Design review of the part built by this model. Coordinates are the model's own, in mm. A direction names the side the tool comes from. Round coordinates to 2 decimals unless told otherwise and drop trailing zeros. Order: outer loops, then holes, each group sorted by start corner. A loop starts at its lowest first (then second) coordinate and runs counter-clockwise, first axis right, second up. Notation, with made-up numbers: (11.5, -18) - (69.5, -18) arc R22 ccw to (69.5, 11) - close; hole circle Ø1 at (17, 29.5). An arc over 180 degrees is marked (long way). Write item = value, one per line.
from build123d import *

# Parameters (mm, degrees)
SKETCH1_W                       = 45.72
SKETCH1_H                       = 60.96
BOSS_EXTRUDE1_DEPTH             = 6.35
SKETCH2_W                       = 7.8600046
SKETCH2_H                       = 60.96
BOSS_EXTRUDE2_DEPTH             = 20.955
LPATTERN1_COUNT                 = 3
LPATTERN1_PITCH                 = 17.018
SKETCH1_3_W                     = 45.72
SKETCH1_3_H                     = 60.96
BOSS_EXTRUDE3_DEPTH             = 2.54
CUT_EXTRUDE1_START              = 14.999995
SKETCH11_W                      = 60.96
SKETCH11_H                      = 14.3449802
CUT_EXTRUDE1_DEPTH              = 17.78
CUT_EXTRUDE2_DEPTH              = 62.358877312
SKETCH17_W                      = 45.72
SKETCH17_H                      = 60.96
BOSS_EXTRUDE4_DEPTH             = 6.985
SKETCH19_W                      = 29.9999908
SKETCH19_H                      = 60.96
BOSS_EXTRUDE5_DEPTH             = 1.0100056
CBORE_FOR_M5_SBHCS2_D           = 5.5
CBORE_FOR_M5_SBHCS2_CBORE_D     = 10.5
CBORE_FOR_M5_SBHCS2_CBORE_DEPTH = 2.75
CUT_EXTRUDE3_DEPTH              = 82.222264916
CUT_EXTRUDE3_DEPTH_BACK         = 82.222264916
SKETCH24_W                      = 5.08
SKETCH24_H                      = 45.72
CUT_EXTRUDE4_DEPTH              = 9.874000032


with BuildPart() as part:
    # Sketch1 → Boss-Extrude1 (new body)
    with BuildSketch(Plane(origin=(0, 0, 0), x_dir=(1, 0, 0), z_dir=(0, 1, 0))):
        Rectangle(SKETCH1_W, SKETCH1_H)
    extrude(amount=BOSS_EXTRUDE1_DEPTH)

    # Sketch2 → Boss-Extrude2 (add)
    with BuildSketch(Plane(origin=(0, 6.35, 0), x_dir=(1, 0, 0), z_dir=(0, 1, 0))):
        with Locations((-18.9299977, 0)):
            Rectangle(SKETCH2_W, SKETCH2_H)
        with Locations((18.9299977, 0)):
            Rectangle(SKETCH2_W, SKETCH2_H)
    extrude(amount=BOSS_EXTRUDE2_DEPTH)

    # Sketch7 → M2 Clearance Hole2 (revolve, cut)
    with BuildSketch(Plane(origin=(22.86, 10.16, 14.9171914), x_dir=(0, 0, -1), z_dir=(0, 1, 0))):
        Polygon((0, 0), (0, 46.441032743), (1.2, 45.72), (1.2, 0), align=None)
    m2_clearance_hole2 = revolve(axis=Axis((29.21, 10.16, 14.9171914), (-1, 0, 0)), mode=Mode.SUBTRACT)

    # LPattern1: M2 Clearance Hole2 ×3
    with Locations(*[(0, 0, -i * LPATTERN1_PITCH) for i in range(1, LPATTERN1_COUNT)]):
        add(m2_clearance_hole2, mode=Mode.SUBTRACT)

    # Sketch1<3> → Boss-Extrude3 (add)
    with BuildSketch(Plane(origin=(0, 0, 0), x_dir=(1, 0, 0), z_dir=(0, 1, 0))):
        Rectangle(SKETCH1_3_W, SKETCH1_3_H)
    extrude(amount=-BOSS_EXTRUDE3_DEPTH)

    # Sketch11 → Cut-Extrude1 (cut, symmetric)
    with BuildSketch(Plane.ZY.offset(-14.9999954).offset(CUT_EXTRUDE1_START)):
        with Locations((0, 20.1325099)):
            Rectangle(SKETCH11_W, SKETCH11_H)
    extrude(amount=CUT_EXTRUDE1_DEPTH, both=True, mode=Mode.SUBTRACT)

    # Sketch12 → Cut-Extrude2 (cut, through all)
    with BuildSketch(Plane(origin=(22.86, 0, 0), x_dir=(0, 0, -1), z_dir=(1, 0, 0))):
        with BuildLine():
            Line((13.105000048, 12.7), (30.48, 12.7))
            Line((30.48, 12.7), (30.48, 27.305))
            Line((30.48, 27.305), (25.661312206, 27.305))
            ThreePointArc((25.661312206, 27.305), (3.474748234, 33.679387055), (13.105000048, 12.7))
        make_face()
    extrude(amount=-CUT_EXTRUDE2_DEPTH, mode=Mode.SUBTRACT)

    # Sketch17 → Boss-Extrude4 (add)
    with BuildSketch(Plane.XZ.offset(2.54)):
        Rectangle(SKETCH17_W, SKETCH17_H)
    extrude(amount=BOSS_EXTRUDE4_DEPTH)

    # Sketch19 → Boss-Extrude5 (add)
    with BuildSketch(Plane(origin=(0, 6.35, 0), x_dir=(1, 0, 0), z_dir=(0, 1, 0))):
        Rectangle(SKETCH19_W, SKETCH19_H)
    extrude(amount=BOSS_EXTRUDE5_DEPTH)

    # CBORE for M5 SBHCS2 (through all)
    with Locations(Plane(origin=(0, 7.3600056, 0), x_dir=(1, 0, 0), z_dir=(0, 1, 0))):
        with Locations((0, -12.7), (0, 19.05)):
            CounterBoreHole(CBORE_FOR_M5_SBHCS2_D / 2, CBORE_FOR_M5_SBHCS2_CBORE_D / 2, CBORE_FOR_M5_SBHCS2_CBORE_DEPTH)

    # Sketch24 → Cut-Extrude3 (cut, two sides: drawn at the far end of the back side and taken through both)
    with BuildSketch(Plane(origin=(31.571183672, -12.7, -14.6188086), x_dir=(0, 0, -1), z_dir=(0, 1, 0)).offset(-CUT_EXTRUDE3_DEPTH_BACK)):
        with Locations((-42.5588086, 31.571183672)):
            Rectangle(SKETCH24_W, SKETCH24_H)
    extrude(amount=CUT_EXTRUDE3_DEPTH + CUT_EXTRUDE3_DEPTH_BACK, mode=Mode.SUBTRACT)

    # Sketch25 → Cut-Extrude4 (cut)
    with BuildSketch(Plane.XY.offset(25.4)):
        Polygon((8.636, -9.525), (8.636, -4.445), (22.86, 9.779), (22.86, -9.525), align=None)
    extrude(amount=-CUT_EXTRUDE4_DEPTH, mode=Mode.SUBTRACT)


solid = part.part
Item 1: Insertion check: P1, Ø12, axis at x = 0, z = 12.7, coming from the +Y side; P2, Ø2.5, axis at y = -6.5, z = 21, coming from the +X side; P3, Ø7, axis at x = 0, z = -19.05, coming from the +Y side. Each pin has a flat end and moves straight along its axis. Give the tip position at first contact, or say it passes through.
Data:
P1 = 7.36
P2 = 8.64
P3 = 4.61
Item 2: The part is to be moulded in two halves that separate along X. For faces 5 (the face through (0.596, -2.556, 15.385)), 6 (the face through (22.86, 9, -3)), 7 (the face through (2, 4.61, 15)), 8 (the face through (20, 27.305, 12)), say which applies: +X half, -X half, draft (parallel to the pull), parting line (faces both ways), or undercut.
Data:
face_5 = undercut
face_6 = +X half
face_7 = undercut
face_8 = draft
Item 3: Take a section at C-C, the plane y = -7. State the section outline as (x, z) points, and give its area (3 significant figures).
Data:
outline = (-22.86, -30.48) - (22.86, -30.48) - (22.86, 15.53) - (8.64, 15.53) - (8.64, 25.4) - (-22.86, 25.4) - close; hole circle Ø5.5 at (0, -19.05); hole circle Ø5.5 at (0, 12.7)
area = 2,370 mm2
Item 4: Take a section at D-D, the plane z = 20.5. State the section outline as (x, y) points (3 decimals).
Data:
outline = (-22.86, -9.525) - (8.636, -9.525) - (8.636, -4.445) - (22.86, 9.779) - (22.86, 27.305) - (17.78, 27.305) - (17.78, 12.96) - (15, 12.96) - (15, 7.36) - (-15, 7.36) - (-15, 12.96) - (-17.78, 12.96) - (-17.78, 27.305) - (-22.86, 27.305) - close
Item 5: Take a section at B-B, the plane z = 12.7. State the section outline as (x, y) points (3 decimals).
Data:
outline = (-22.86, -9.525) - (-2.75, -9.525) - (-2.75, 4.61) - (-5.25, 4.61) - (-5.25, 7.36) - (-15, 7.36) - (-15, 12.96) - (-17.78, 12.96) - (-17.78, 27.305) - (-22.86, 27.305) - close; (2.75, -9.525) - (22.86, -9.525) - (22.86, 27.305) - (17.78, 27.305) - (17.78, 12.96) - (15, 12.96) - (15, 7.36) - (5.25, 7.36) - (5.25, 4.61) - (2.75, 4.61) - close
Item 6: For faces 1 (the face through (8.636, -7, 21)), 2 (the face through (-19.748, 17.237, -3.376)), 3 (the face through (15, 8, -2)), 4 (the face through (-19, 12.7, -22)), list the 3-axis set-ups (+Z, -Z, +X, -X, +Y, -Y) from which the entire face can be reached by the end or side of a thin tool; tool diameter is ignored.
Data:
face_1 = +Z, +X, -Y
face_2 = -Z, +X, -X
face_3 = +Z, -Z, +Y
face_4 = -Z, +X, -X, +Y
Item 7: For line 1 along Z through (x, y) = (-17, 10.16); line 2 along Z through (x, y) = (0, 6); line 3 along X through (y, z) = (16, 19), list the stretches that pass through material, from the lowest coordinate up. Write a range as [from, to].
Data:
line_1 = [-30.48, -20.32], [-17.92, -3.3], [-0.9, 13.72], [16.12, 25.4]
line_2 = [-30.48, -24.3], [-13.8, 7.45], [17.95, 25.4]
line_3 = [-22.86, -17.78], [17.78, 22.86]
Item 8: Take a section at A-A, the plane x = 0. State the section outline as (y, z) points (3 decimals), and give its area (3 significant figures).
Data:
outline = (-9.525, -30.48) - (7.36, -30.48) - (7.36, -24.3) - (4.61, -24.3) - (4.61, -21.8) - (-9.525, -21.8) - close; (-9.525, -16.3) - (4.61, -16.3) - (4.61, -13.8) - (7.36, -13.8) - (7.36, 7.45) - (4.61, 7.45) - (4.61, 9.95) - (-9.525, 9.95) - close; (-9.525, 15.45) - (4.61, 15.45) - (4.61, 17.95) - (7.36, 17.95) - (7.36, 25.4) - (-9.525, 25.4) - close
area = 730 mm2
